from build123d import *

# Parameters (mm, degrees)
F0_W     = 300
F0_H     = 150
F1_DEPTH = 12
F2_R     = 4.5
F3_DEPTH = 25
F4_R     = 4.5
F5_DEPTH = 25


with BuildPart() as f1:
    # F0 (on Top) → F1 (new body)
    with BuildSketch(Plane.XY):
        Rectangle(F0_W, F0_H)
    extrude(amount=F1_DEPTH)

    # F2 (on face) → F3 (join)
    with BuildSketch(Plane.YZ.offset(150)):
        with Locations((-63, 6)):
            Circle(F2_R)
        with Locations((63, 6)):
            Circle(F2_R)
    extrude(amount=F3_DEPTH)

    # F4 (on face) → F5 (join)
    with BuildSketch(Plane(origin=(-150, 0, 0), x_dir=(0, -1, 0), z_dir=(-1, 0, 0))):
        with Locations((-63, 6)):
            Circle(F4_R)
        with Locations((63, 6)):
            Circle(F4_R)
    extrude(amount=F5_DEPTH)


solid = f1.part
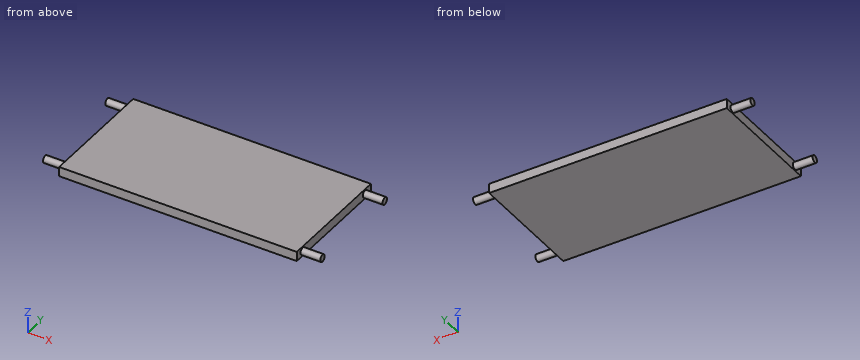
The model under review builds one solid part; all positions refer to its coordinate system, in mm. Round coordinates to 2 decimals unless told otherwise and drop trailing zeros. Loops run counter-clockwise (first coordinate to the right, second up) from the corner with the lowest first, then second, coordinate; pieces in that order, holes last. Notation, with made-up numbers: (26, 35.25) -> (32, 35.25) arc R6 ccw to (32, 39.25) -> close; hole circle Ø5 at (40.5, -27). An arc over 180 degrees is marked (long way). One line per question, with ' | ' between items. Start each with the question number.
Item 1: Wall thickness on line 1 along Z through (x, y) = (-159, 62.5); line 2 along X through (y, z) = (42.5, 9.5); line 3 along Y through (x, z) = (158.5, 2.25): over which ranges is each line inside the solid? List them lowest first. Write a range as [from, to].
Item 2: Add section B-B, the plane z = 6. Write out the cut boundary in (x, y).
Item 3: Add section C-C, the plane y = -15.5. Write out the cut boundary in (x, z), then the cut area to 3 significant figures.
Item 4: For pin 1 (3.5 mm diameter, centred on y = 25.5, z = 3, fed in from +X); pin 2 (5 mm diameter, centred on y = -49.5, z = 10.5, fed in from -X), all flat-tipped, find the tip position at first contact; note any pin that passes through.
Item 5: Add section A-A, the plane y = -63. Write out the cut boundary in (x, z).
Return value:
1) line 1: z = [1.53, 10.47] | line 2: x = [-150, 150] | line 3: y = [-65.49, -60.51], [60.51, 65.49]
2) outline: (-175, -67.5) -> (-150, -67.5) -> (-150, -75) -> (150, -75) -> (150, -67.5) -> (175, -67.5) -> (175, -58.5) -> (150, -58.5) -> (150, 58.5) -> (175, 58.5) -> (175, 67.5) -> (150, 67.5) -> (150, 75) -> (-150, 75) -> (-150, 67.5) -> (-175, 67.5) -> (-175, 58.5) -> (-150, 58.5) -> (-150, -58.5) -> (-175, -58.5) -> close
3) outline: (-150, 0) -> (150, 0) -> (150, 12) -> (-150, 12) -> close | area: 3,600 mm2
4) pin 1: stops at x = 150 | pin 2: stops at x = -150
5) outline: (-175, 1.5) -> (-150, 1.5) -> (-150, 0) -> (150, 0) -> (150, 1.5) -> (175, 1.5) -> (175, 10.5) -> (150, 10.5) -> (150, 12) -> (-150, 12) -> (-150, 10.5) -> (-175, 10.5) -> close
